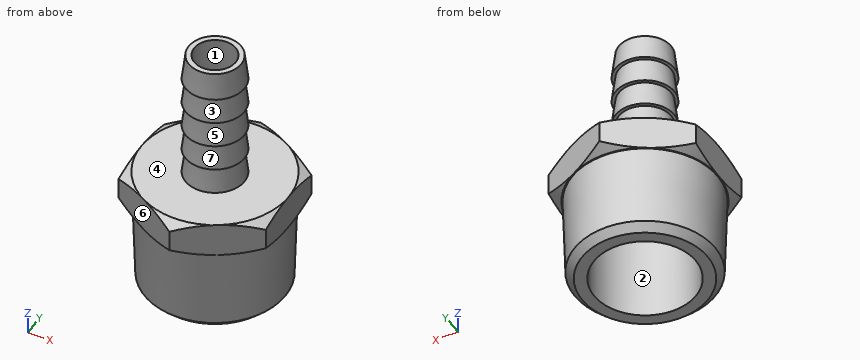
```python
from build123d import *

# Parameters (mm, degrees)
LPATTERN1_COUNT     = 5
LPATTERN1_PITCH     = 4.9
BOSS_EXTRUDE1_START = -7.3
BOSS_EXTRUDE1_DEPTH = 6.3
SKETCH5_OUTSIDE_W   = 153.692
SKETCH5_OUTSIDE_H   = 157.868
SKETCH5_OUTSIDE_R   = 13.5
CUT_EXTRUDE1_DEPTH  = 33.023428923
CUT_EXTRUDE1_DRAFT  = -60
SKETCH6_OUTSIDE_W   = 171.16
SKETCH6_OUTSIDE_H   = 175.336
SKETCH6_OUTSIDE_R   = 13.5
CUT_EXTRUDE2_DEPTH  = 38.066022177
CUT_EXTRUDE2_DRAFT  = -60


with BuildPart() as part:
    # Sketch2 → Revolve2 (revolve)
    with BuildSketch(Plane(origin=(0, 0, 0), x_dir=(0, 0, -1), z_dir=(1, 0, 0)), mode=Mode.PRIVATE) as revolve2_sk:
        Polygon((-23.5, 4.8), (-18.6, 5.4), (-18.6, 0), (-23.5, 0), align=None)
    revolve(revolve2_sk.sketch.rotate(Axis((0, 0, 23.5), (0, 0, -1)), 180), axis=Axis((0, 0, 23.5), (0, 0, -1)))


with BuildPart() as lpattern1_1:
    # LPattern1: pattern copy
    add(part.part.moved(Location(Vector(0, 0, -1) * (1 * LPATTERN1_PITCH))))


with BuildPart() as lpattern1_2:
    # LPattern1: pattern copy
    add(part.part.moved(Location(Vector(0, 0, -1) * (2 * LPATTERN1_PITCH))))


with BuildPart() as lpattern1_3:
    # LPattern1: pattern copy
    add(part.part.moved(Location(Vector(0, 0, -1) * (3 * LPATTERN1_PITCH))))


with BuildPart() as lpattern1_4:
    # LPattern1: pattern copy
    add(part.part.moved(Location(Vector(0, 0, -1) * (4 * LPATTERN1_PITCH))))


with BuildPart() as body_6:
    # Sketch3 → Boss-Extrude1 (new body)
    with BuildSketch(Plane.XY.offset(BOSS_EXTRUDE1_START)):
        Polygon((0, 15.588457268), (-13.5, 7.794228634), (-13.5, -7.794228634), (0, -15.588457268), (13.5, -7.794228634), (13.5, 7.794228634), align=None)
    extrude(amount=BOSS_EXTRUDE1_DEPTH)


with BuildPart() as cut_extrude1_tool:
    # Sketch5 outside → Cut-Extrude1 (with draft: the straight prism first)
    with BuildSketch(Plane.XY.offset(-1)):
        Rectangle(SKETCH5_OUTSIDE_W, SKETCH5_OUTSIDE_H)
        Circle(SKETCH5_OUTSIDE_R, mode=Mode.SUBTRACT)
    extrude(amount=-CUT_EXTRUDE1_DEPTH)
    # Cut-Extrude1: the draft: its side faces are tilted about the plane it starts from
    cut_extrude1_sides = [cut_extrude1_tool.faces().sort_by_distance(p)[0] for p in [
        (0, -78.934, -17.511714462),
        (76.846, 0, -17.511714462),
        (0, 78.934, -17.511714462),
        (-76.846, 0, -17.511714462),
        (-13.5, 0, -17.511714462),
    ]]
    draft(cut_extrude1_sides, Plane.XY.offset(-1), CUT_EXTRUDE1_DRAFT)


with BuildPart() as body_6_1:
    add(body_6.part)

    # Cut-Extrude1: cut by cut_extrude1_tool
    add(cut_extrude1_tool.part, mode=Mode.SUBTRACT)


with BuildPart() as cut_extrude2_tool:
    # Sketch6 outside → Cut-Extrude2 (with draft: the straight prism first)
    with BuildSketch(Plane(origin=(0, 0, -7.3), x_dir=(-1, 0, 0), z_dir=(0, 0, -1))):
        Rectangle(SKETCH6_OUTSIDE_W, SKETCH6_OUTSIDE_H)
        Circle(SKETCH6_OUTSIDE_R, mode=Mode.SUBTRACT)
    extrude(amount=-CUT_EXTRUDE2_DEPTH)
    # Cut-Extrude2: the draft: its side faces are tilted about the plane it starts from
    cut_extrude2_sides = [cut_extrude2_tool.faces().sort_by_distance(p)[0] for p in [
        (0, -87.668, 11.733011088),
        (-85.58, 0, 11.733011088),
        (0, 87.668, 11.733011088),
        (85.58, 0, 11.733011088),
        (13.5, 0, 11.733011088),
    ]]
    draft(cut_extrude2_sides, Plane(origin=(0, 0, -7.3), x_dir=(-1, 0, 0), z_dir=(0, 0, -1)), CUT_EXTRUDE2_DRAFT)


with BuildPart() as body_6_2:
    add(body_6_1.part)

    # Cut-Extrude2: cut by cut_extrude2_tool
    add(cut_extrude2_tool.part, mode=Mode.SUBTRACT)


with BuildPart() as part_1:
    add(part.part)

    add(lpattern1_1.part)  # Revolve1 merges LPattern1_1

    add(lpattern1_2.part)  # Revolve1 merges LPattern1_2

    add(lpattern1_3.part)  # Revolve1 merges LPattern1_3

    add(lpattern1_4.part)  # Revolve1 merges LPattern1_4

    add(body_6_2.part)  # Revolve1 merges body 6
    # Sketch4 → Revolve1 (revolve)
    with BuildSketch(Plane(origin=(0, 0, 0), x_dir=(0, 0, -1), z_dir=(1, 0, 0)), mode=Mode.PRIVATE) as revolve1_sk:
        Polygon((-23.5, 4.8), (7.3, 4.8), (7.3, 13.335), (22.139285714, 12.872977456), (23.5, 11.51226317), (23.5, 0), (-23.5, 0), align=None)
    revolve(revolve1_sk.sketch.rotate(Axis((0, 0, 23.5), (0, 0, -1)), 180), axis=Axis((0, 0, 23.5), (0, 0, -1)))

    # Sketch7 → Cut-Revolve1 (revolve, cut)
    with BuildSketch(Plane(origin=(0, 0, 0), x_dir=(0, 0, -1), z_dir=(1, 0, 0)), mode=Mode.PRIVATE) as cut_revolve1_sk:
        Polygon((-23.5, 0), (-23.5, 3.8), (4.15, 3.8), (4.15, 9.3345), (23.5, 9.3345), (23.5, 0), align=None)
    revolve(cut_revolve1_sk.sketch.rotate(Axis((0, 0, 23.5), (0, 0, -1)), 180), axis=Axis((0, 0, 23.5), (0, 0, -1)), mode=Mode.SUBTRACT)


solid = part_1.part
```
Build history of the part. All positions in model axes, mm. Face numbers are marked on the shaded views. A direction names the side the tool comes from. Coordinates: 2 decimals unless noted, no trailing zeros. Write each loop counter-clockwise with the first axis right and the second up, starting at its lowest first coordinate (ties: lowest second). Pieces come first, ordered by that corner, then holes.
1. Band-saw the part on B-B, the plane z = 13. Give the cut face in (x, y).
Answer block:
outline: circle Ø9.77 at (0, 0); hole circle Ø7.6 at (0, 0)
2. 3-axis set-ups, long thin cutter, end or side, ignore diameter. For the marked faces 1, 2 and 3: which of +Z, -Z, +X, -X, +Y, -Y reach the whole face in a straight line?
Answer block:
face 1: +Z, -Z
face 2: -Z
face 3: none
3. Drop flat-ended pins along their axis: pin 1 (9.5 mm diameter, centred on x = 4, y = 1, fed in from -Z); pin 2 (3 mm diameter, centred on y = -4, z = 13, fed in from -X); pin 3 (8.5 mm diameter, centred on x = 0, y = 0, fed in from -Z); pin 4 (3 mm diameter, centred on x = -0.5, y = 0, fed in from -Z). Give the stop position or say it passes through.
Answer block:
pin 1: stops at z = -4.15
pin 2: stops at x = -4.69
pin 3: stops at z = -4.15
pin 4: passes through
4. Drill centre lines: probe 1 along X at (y, z) = (0, 4); probe 2 along X at (y, z) = (-5.5, -20); probe 3 along Z at (x, y) = (-5.75, 6.5). Where is each one in solid material? Low to high.
Answer block:
probe 1: x = -5.39 to -3.8, 3.8 to 5.39
probe 2: x = -11.71 to -7.54, 7.54 to 11.71
probe 3: z = -4.15 to -1
5. Band-saw the part on A-A, the plane z = -10. Give the cut face in (x, y).
Answer block:
outline: circle Ø26.5 at (0, 0); hole circle Ø18.67 at (0, 0)
6. Pull direction Z, two halves, no side cores. Call the marked faces 4, 5, 6 and 7: released by +Z, released by -Z, zero draft, split by the parting line, or undercut.
Answer block:
face 4: released by +Z
face 5: undercut
face 6: zero draft
face 7: undercut
